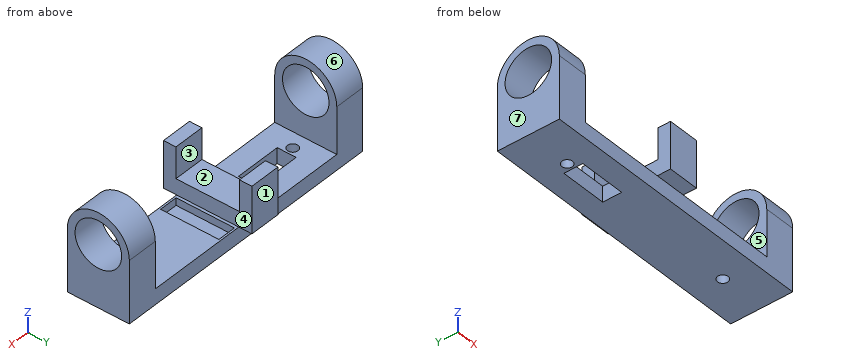
```python
from build123d import *

# Parameters (mm, degrees)
ESQUISSE1_W             = 90
ESQUISSE1_H             = 20
BOSS_EXTRU_1_DEPTH      = 5
ESQUISSE2_W             = 10
ESQUISSE2_H             = 20
BOSS_EXTRU_2_DEPTH      = 30
ESQUISSE3_R             = 7.5
ENL_V_MAT_EXTRU_1_DEPTH = 10
ESQUISSE5_W             = 6
ESQUISSE5_H             = 18.8
ENL_V_MAT_EXTRU_2_DEPTH = 2.4
ESQUISSE10_W            = 15
ESQUISSE10_H            = 6.1
ENL_V_MAT_EXTRU_4_DEPTH = 5
ESQUISSE11_R            = 1
ENL_V_MAT_EXTRU_5_DEPTH = 10
D_GAGEMENT_M31_D        = 3.4
ESQUISSE14_W            = 10
ESQUISSE14_H            = 28.5
BOSS_EXTRU_3_DEPTH      = 5
ESQUISSE16_W            = 10
ESQUISSE16_H            = 4
BOSS_EXTRU_4_DEPTH      = 10


with BuildPart() as part:
    # Esquisse1 → Boss.-Extru.1 (new body)
    with BuildSketch(Plane.XY):
        with Locations((45, 10)):
            Rectangle(ESQUISSE1_W, ESQUISSE1_H)
    extrude(amount=BOSS_EXTRU_1_DEPTH)

    # Esquisse2 → Boss.-Extru.2 (add)
    with BuildSketch(Plane.XY.offset(5)):
        with Locations((5, 10)):
            Rectangle(ESQUISSE2_W, ESQUISSE2_H)
    boss_extru_2 = extrude(amount=BOSS_EXTRU_2_DEPTH)

    # Esquisse3 → Enlèv. mat.-Extru.1 (cut)
    with BuildSketch(Plane.ZY):
        with Locations((20, 10)):
            Circle(ESQUISSE3_R)
        with BuildLine():
            Line((35, 20), (20, 20))
            ThreePointArc((20, 20), (30, 10), (20, 0))
            Line((20, 0), (35, 0))
            Line((35, 0), (35, 20))
        make_face()
    enl_v_mat_extru_1 = extrude(amount=-ENL_V_MAT_EXTRU_1_DEPTH, mode=Mode.SUBTRACT)

    # Symétrie1: Boss.-Extru.2, Enlèv. mat.-Extru.1 across plane
    add(boss_extru_2.mirror(Plane(origin=(45, 0, 0), x_dir=(0, 0, 1), z_dir=(1, 0, 0))))
    add(enl_v_mat_extru_1.mirror(Plane(origin=(45, 0, 0), x_dir=(0, 0, 1), z_dir=(1, 0, 0))), mode=Mode.SUBTRACT)

    # Esquisse5 → Enlèv. mat.-Extru.2 (cut)
    with BuildSketch(Plane.XY.offset(5)):
        with Locations((51.75, 10)):
            Rectangle(ESQUISSE5_W, ESQUISSE5_H)
    extrude(amount=-ENL_V_MAT_EXTRU_2_DEPTH, mode=Mode.SUBTRACT)

    # Esquisse10 → Enlèv. mat.-Extru.4 (cut)
    with BuildSketch(Plane.XY.offset(5)):
        with Locations((24.85, 10)):
            Rectangle(ESQUISSE10_W, ESQUISSE10_H)
    extrude(amount=-ENL_V_MAT_EXTRU_4_DEPTH, mode=Mode.SUBTRACT)

    # Esquisse11 → Enlèv. mat.-Extru.5 (cut)
    with BuildSketch(Plane.XY.offset(5)):
        with Locations((15, 10)):
            Circle(ESQUISSE11_R)
        with Locations((75, 10)):
            Circle(ESQUISSE11_R)
    extrude(amount=-ENL_V_MAT_EXTRU_5_DEPTH, mode=Mode.SUBTRACT)

    # Dégagement M31 (through all)
    with Locations(Plane.XY.offset(5)):
        with Locations((15, 10), (75, 10)):
            Hole(D_GAGEMENT_M31_D / 2)

    # Esquisse14 → Boss.-Extru.3 (add)
    with BuildSketch(Plane.XY.offset(5)):
        with Locations((42.803073496, 10.001209338)):
            Rectangle(ESQUISSE14_W, ESQUISSE14_H)
    extrude(amount=BOSS_EXTRU_3_DEPTH)

    # Esquisse16 → Boss.-Extru.4 (add)
    with BuildSketch(Plane.XY.offset(10)):
        with Locations((42.803073496, 22.251209338)):
            Rectangle(ESQUISSE16_W, ESQUISSE16_H)
        with Locations((42.803073496, -2.248790662)):
            Rectangle(ESQUISSE16_W, ESQUISSE16_H)
    extrude(amount=BOSS_EXTRU_4_DEPTH)


solid = part.part
```
Read the model definition and answer for the solid it produces. Units are mm, in the model's axes. Face numbers are marked on the shaded views. A direction names the side the tool comes from. Coordinates: 2 decimals unless noted, no trailing zeros. Loops run counter-clockwise (first coordinate to the right, second up) from the corner with the lowest first, then second, coordinate; pieces in that order, holes last. Notation, with made-up numbers: (34, 45) -> (78, 45) arc R17 cw to (78, 73) -> close; hole circle Ø8 at (74.5, 83). An arc over 180 degrees is marked (long way). Return JSON: item names as keys, results as strings.
Item 1: Find section B-B (z = 11.5). Determine the outline of the cut face in (x, y).
Answers:
{"outline": "(0, 0) -> (10, 0) -> (10, 20) -> (0, 20) -> close; (37.8, -4.25) -> (47.8, -4.25) -> (47.8, -0.25) -> (37.8, -0.25) -> close; (37.8, 20.25) -> (47.8, 20.25) -> (47.8, 24.25) -> (37.8, 24.25) -> close; (80, 0) -> (90, 0) -> (90, 20) -> (80, 20) -> close"}
Item 2: Flat-ended cylindrical pins translate along their axes: P1, Ø12, axis at x = 74.5, y = 14, coming from the +Z side; P2, Ø2.5, axis at x = 53, z = 4.5, coming from the -Y side; P3, Ø1.3, axis at x = 44, y = 22.5, coming from the -Z side. Find the tip coordinate at first contact, or state that the pin passes through.
Answers:
{"P1": "stops at z = 29.87", "P2": "stops at y = 0", "P3": "stops at z = 5"}
Item 3: Find section D-D (z = 7.25). Determine the outline of the cut face in (x, y), plus the area to 3 significant figures.
Answers:
{"outline": "(0, 0) -> (10, 0) -> (10, 20) -> (0, 20) -> close; (37.8, -4.25) -> (47.8, -4.25) -> (47.8, 24.25) -> (37.8, 24.25) -> close; (80, 0) -> (90, 0) -> (90, 20) -> (80, 20) -> close", "area": "685 mm2"}
Item 4: For a pull along X with two mould halves and no side action, classify the marked faces 5, 6 and 7 as +X half, -X half, draft (parallel to the pull), parting line (faces both ways), or undercut.
Answers:
{"face 5": "undercut", "face 6": "draft", "face 7": "-X half"}
Item 5: Find section C-C (y = 4). Determine the outline of the cut face in (x, z), plus the area to 3 significant figures.
Answers:
{"outline": "(0, 0) -> (90, 0) -> (90, 15.5) -> (80, 15.5) -> (80, 5) -> (54.75, 5) -> (54.75, 2.6) -> (48.75, 2.6) -> (48.75, 5) -> (47.8, 5) -> (47.8, 10) -> (37.8, 10) -> (37.8, 5) -> (10, 5) -> (10, 15.5) -> (0, 15.5) -> close; (0, 24.5) -> (10, 24.5) -> (10, 28) -> (0, 28) -> close; (80, 24.5) -> (90, 24.5) -> (90, 28) -> (80, 28) -> close", "area": "766 mm2"}
Item 6: For the marked faces 1, 2, 3 and 4, determine the directions among +Z, -Z, +X, -X, +Y, -Y from which every point of the face is accessible in a straight line to the end or side of a thin tool.
Answers:
{"face 1": "+Z, -Z, +X, -X, +Y", "face 2": "+Z", "face 3": "+Z, +X, -X", "face 4": "+Z, +Y, -Y"}
Item 7: Find the intervals of material crossed by probe 1 along X at (y, z) = (10.75, 9.5); probe 2 along Y at (x, z) = (30, 2); probe 3 along Y at (x, z) = (85.5, 20), in increasing order.
Answers:
{"probe 1": "x = 0 to 10, 37.8 to 47.8, 80 to 90", "probe 2": "y = 0 to 6.95, 13.05 to 20", "probe 3": "y = 0 to 2.5, 17.5 to 20"}
Item 8: Find section A-A (x = 15). Determine the outline of the cut face in (y, z).
Answers:
{"outline": "(0, 0) -> (8.3, 0) -> (8.3, 5) -> (0, 5) -> close; (11.7, 0) -> (20, 0) -> (20, 5) -> (11.7, 5) -> close"}
